```python
from build123d import *

# Parameters (mm, degrees)
SKETCH_1_R      = 48
SLEEVE_DEPTH    = 8
SKETCH_2_R      = 40
BORE_DEPTH      = 69.352029963
ROUNDED_EDGES_R = 1.5


with BuildPart() as part:
    # 草图1 → Sleeve (new body)
    with BuildSketch(Plane.XY):
        Circle(SKETCH_1_R)
    extrude(amount=SLEEVE_DEPTH)

    # 草图2 → Bore (cut, through all)
    with BuildSketch(Plane.XY.offset(8)):
        Circle(SKETCH_2_R)
    extrude(amount=-BORE_DEPTH, mode=Mode.SUBTRACT)

    # Rounded_edges
    rounded_edges_edges = [part.edges().sort_by_distance(p)[0] for p in [
        (-48, 0, 0),
        (-48, 0, 8),
        (-40, 0, 0),
        (-40, 0, 8),
    ]]
    fillet(rounded_edges_edges, radius=ROUNDED_EDGES_R)


solid = part.part
```
The model under review builds one solid part; all positions refer to its coordinate system, in mm. Coordinates: 2 decimals unless noted, no trailing zeros. Order: outer loops, then holes, each group sorted by start corner. A loop starts at its lowest first (then second) coordinate and runs counter-clockwise, first axis right, second up. Notation, with made-up numbers: M 14.5,62.25 L 54.5,62.25 A6 ccw 54.5,73.25 Z; hole C 32,45.5 d3. An arc over 180 degrees is marked long. One line per question, with ' | ' between items.
(1) Add section C-C, the plane z = 4.25. Write out the cut boundary in (x, y).
Geometry results:
outline: C 0,0 d96; hole C 0,0 d80
(2) For probe 1 along Y at (x, z) = (0, 5.4); probe 2 along Y at (x, z) = (-9, 1.25); probe 3 along X at (y, z) = (13, 6), list the stretches that pass through material, from the lowest coordinate up. Write a range as from..to.
Geometry results:
probe 1: y = -48..-40, 40..48 | probe 2: y = -47.13..-39, 39..47.13 | probe 3: x = -46.21..-37.83, 37.83..46.21
(3) Add section A-A, the plane y = 0. Write out the cut boundary in (x, z), then the cut area to 3 significant figures.
Geometry results:
outline: M -48,1.5 A1.5 ccw -46.5,0 L -41.5,0 A1.5 ccw -40,1.5 L -40,6.5 A1.5 ccw -41.5,8 L -46.5,8 A1.5 ccw -48,6.5 Z; M 40,1.5 A1.5 ccw 41.5,0 L 46.5,0 A1.5 ccw 48,1.5 L 48,6.5 A1.5 ccw 46.5,8 L 41.5,8 A1.5 ccw 40,6.5 Z | area: 124 mm²
(4) Insertion check: pin 1 (1.5 mm diameter, centred on x = -35, z = 2.5, fed in from -Y); pin 2 (1 mm diameter, centred on x = 27.5, z = 3.5, fed in from -Y). Each pin has a flat end and moves straight along its axis. Give the tip position at first contact, or say it passes through.
Geometry results:
pin 1: stops at y = -33.63 | pin 2: stops at y = -39.69
